from build123d import *

# Parameters (mm, degrees)
SALIENTE_EXTRUIR2_DEPTH      = 4.6
SALIENTE_EXTRUIR3_DEPTH      = 5.1
SALIENTE_EXTRUIR3_DEPTH_BACK = 4.6
CROQUIS2_R                   = 4.75
CROQUIS4_R                   = 5.025
SALIENTE_EXTRUIR4_DEPTH      = 1.5
CROQUIS6_R                   = 3.75
SALIENTE_EXTRUIR5_DEPTH      = 2.3
CROQUIS7_R                   = 4.5
SALIENTE_EXTRUIR6_DEPTH      = 2.8


with BuildPart() as part:
    # Croquis1 → Saliente-Extruir2 (new body)
    # profile 1 of 5: a face of its own
    with BuildSketch(Plane(origin=(0, 0, 0), x_dir=(1, 0, 0), z_dir=(0, 1, 0))):
        with BuildLine():
            ThreePointArc((6.5, 9.5), (8.621320344, 8.621320344), (9.5, 6.5))
            Line((9.5, 6.5), (9.5, -6.5))
            ThreePointArc((9.5, -6.5), (8.621320344, -8.621320344), (6.5, -9.5))
            Line((6.5, -9.5), (-6.5, -9.5))
            ThreePointArc((-6.5, -9.5), (-8.621320344, -8.621320344), (-9.5, -6.5))
            Line((-9.5, -6.5), (-9.5, 6.5))
            ThreePointArc((-9.5, 6.5), (-8.621320344, 8.621320344), (-6.5, 9.5))
            Line((-6.5, 9.5), (6.5, 9.5))
        make_face()
        with BuildLine():
            ThreePointArc((4.25, -4.75), (4.603553391, -4.603553391), (4.75, -4.25))
            Line((4.75, -4.25), (4.75, 4.25))
            ThreePointArc((4.75, 4.25), (4.603553391, 4.603553391), (4.25, 4.75))
            Line((4.25, 4.75), (-4.25, 4.75))
            ThreePointArc((-4.25, 4.75), (-4.603553391, 4.603553391), (-4.75, 4.25))
            Line((-4.75, 4.25), (-4.75, -4.25))
            ThreePointArc((-4.75, -4.25), (-4.603553391, -4.603553391), (-4.25, -4.75))
            Line((-4.25, -4.75), (4.25, -4.75))
        make_face(mode=Mode.SUBTRACT)
    # profile 2 of 5: a face of its own
    with BuildSketch(Plane(origin=(0, 0, 0), x_dir=(1, 0, 0), z_dir=(0, 1, 0))):
        with BuildLine():
            ThreePointArc((0, -4.75), (-3.358757211, -3.358757211), (-4.75, 0))
            Line((-4.75, 0), (-4.75, -4.25))
            ThreePointArc((-4.75, -4.25), (-4.603553391, -4.603553391), (-4.25, -4.75))
            Line((-4.25, -4.75), (0, -4.75))
        make_face()
    # profile 3 of 5: a face of its own
    with BuildSketch(Plane(origin=(0, 0, 0), x_dir=(1, 0, 0), z_dir=(0, 1, 0))):
        with BuildLine():
            Line((4.75, -4.25), (4.75, 0))
            ThreePointArc((4.75, 0), (3.358757211, -3.358757211), (0, -4.75))
            Line((0, -4.75), (4.25, -4.75))
            ThreePointArc((4.25, -4.75), (4.603553391, -4.603553391), (4.75, -4.25))
        make_face()
    # profile 4 of 5: a face of its own
    with BuildSketch(Plane(origin=(0, 0, 0), x_dir=(1, 0, 0), z_dir=(0, 1, 0))):
        with BuildLine():
            Line((4.25, 4.75), (0, 4.75))
            ThreePointArc((0, 4.75), (3.358757211, 3.358757211), (4.75, 0))
            Line((4.75, 0), (4.75, 4.25))
            ThreePointArc((4.75, 4.25), (4.603553391, 4.603553391), (4.25, 4.75))
        make_face()
    # profile 5 of 5: a face of its own
    with BuildSketch(Plane(origin=(0, 0, 0), x_dir=(1, 0, 0), z_dir=(0, 1, 0))):
        with BuildLine():
            Line((0, 4.75), (-4.25, 4.75))
            ThreePointArc((-4.25, 4.75), (-4.603553391, 4.603553391), (-4.75, 4.25))
            Line((-4.75, 4.25), (-4.75, 0))
            ThreePointArc((-4.75, 0), (-3.358757211, 3.358757211), (0, 4.75))
        make_face()
    extrude(amount=SALIENTE_EXTRUIR2_DEPTH)

    # Croquis2 → Saliente-Extruir3 (add, two sides: drawn at the far end of the back side and taken through both)
    with BuildSketch(Plane(origin=(0, 4.6, 0), x_dir=(1, 0, 0), z_dir=(0, 1, 0)).offset(-SALIENTE_EXTRUIR3_DEPTH_BACK)):
        with Locations(Location((0, 0, 0), (0, 0, 270))):
            Circle(CROQUIS2_R)
    extrude(amount=SALIENTE_EXTRUIR3_DEPTH + SALIENTE_EXTRUIR3_DEPTH_BACK)

    # Croquis4 → Saliente-Extruir4 (add)
    with BuildSketch(Plane(origin=(0, 9.7, 0), x_dir=(1, 0, 0), z_dir=(0, 1, 0))):
        with Locations(Location((0, 0, 0), (0, 0, 270))):
            Circle(CROQUIS4_R)
    extrude(amount=SALIENTE_EXTRUIR4_DEPTH)

    # Croquis6 → Saliente-Extruir5 (add)
    with BuildSketch(Plane(origin=(0, 11.2, 0), x_dir=(1, 0, 0), z_dir=(0, 1, 0))):
        with Locations(Location((0, 0, 0), (0, 0, 270))):
            Circle(CROQUIS6_R)
    extrude(amount=SALIENTE_EXTRUIR5_DEPTH)

    # Croquis7 → Saliente-Extruir6 (add)
    with BuildSketch(Plane(origin=(0, 13.5, 0), x_dir=(1, 0, 0), z_dir=(0, 1, 0))):
        with Locations(Location((0, 0, 0), (0, 0, 270))):
            Circle(CROQUIS7_R)
    extrude(amount=SALIENTE_EXTRUIR6_DEPTH)


solid = part.part
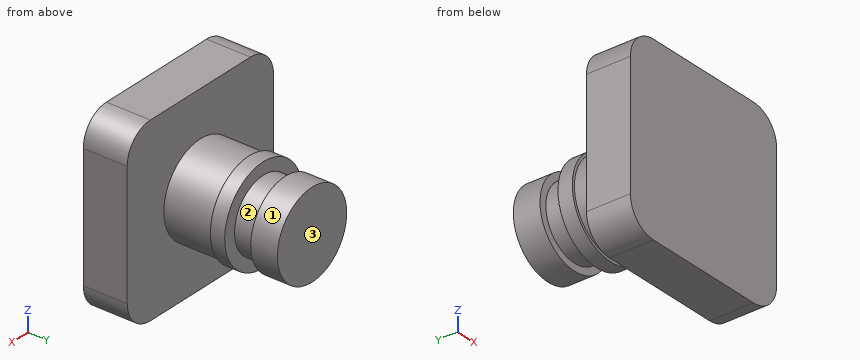
Geometry: final body of the model. Coordinates: model frame, mm. Face numbers are marked on the shaded views. A direction names the side the tool comes from. Give positions to 0.01 mm unless a question says otherwise; leave off trailing zeros. Write each loop counter-clockwise with the first axis right and the second up, starting at its lowest first coordinate (ties: lowest second). Pieces come first, ordered by that corner, then holes. Notation, with made-up numbers: (-29.5, 74.25) - (-19.5, 74.25) arc R19 ccw to (-19.5, 90.25) - close; hole circle Ø6 at (23, 73). An arc over 180 degrees is marked (long way). Return JSON: item names as keys, results as strings. Group by question number.
1) Set-up query: the marked faces 1, 2 and 3. Return all of +Z, -Z, +X, -X, +Y, -Y with unobstructed straight access to the full face (end or side cutting, diameter ignored); none if empty.
2) Line query: line 1 (Y direction, x = -3, z = -3.75); line 2 (Y direction, x = -3.5, z = 2.25); line 3 (Y direction, x = 2.25, z = 5.75). Output: solid intervals per line, ascending.
3) Section A-A on x = 0. Return the cut outline in (y, z) (3 decimals).
4) First-contact query: P1, Ø8, axis at x = -7.5, z = -7, coming from the +Y side; P2, Ø1.5, axis at y = 11, z = 2.5, coming from the +X side; P3, Ø2, axis at x = 5, y = 11.5, coming from the -Z side. Flat tips, straight axial feed; report the tip coordinate or a pass-through.
5) Section B-B on z = 0. Return the cut outline in (x, y) (3 decimals).
6) Section C-C on y = 6.25. Return the cut outline in (x, z), plus the area to 3 significant figures.
7) Section D-D on z = 8.5. Return the cut outline in (x, y), plus the area to 3 significant figures.
Filled in:
{
 "1": {"face 1": "+Y", "face 2": "none", "face 3": "+Z, -Z, +X, -X, +Y"},
 "2": {"line 1": "y = 0 to 4.6, 9.7 to 11.2", "line 2": "y = 0 to 11.2, 13.5 to 16.3", "line 3": "y = 0 to 4.6"},
 "3": {"outline": "(0, -9.5) - (4.6, -9.5) - (4.6, -4.75) - (9.7, -4.75) - (9.7, -5.025) - (11.2, -5.025) - (11.2, -3.75) - (13.5, -3.75) - (13.5, -4.5) - (16.3, -4.5) - (16.3, 4.5) - (13.5, 4.5) - (13.5, 3.75) - (11.2, 3.75) - (11.2, 5.025) - (9.7, 5.025) - (9.7, 4.75) - (4.6, 4.75) - (4.6, 9.5) - (0, 9.5) - close"},
 "4": {"P1": "stops at y = 4.6", "P2": "stops at x = 4.71", "P3": "stops at z = -2.98"},
 "5": {"outline": "(-9.5, 0) - (9.5, 0) - (9.5, 4.6) - (4.75, 4.6) - (4.75, 9.7) - (5.025, 9.7) - (5.025, 11.2) - (3.75, 11.2) - (3.75, 13.5) - (4.5, 13.5) - (4.5, 16.3) - (-4.5, 16.3) - (-4.5, 13.5) - (-3.75, 13.5) - (-3.75, 11.2) - (-5.025, 11.2) - (-5.025, 9.7) - (-4.75, 9.7) - (-4.75, 4.6) - (-9.5, 4.6) - close"},
 "6": {"outline": "circle Ø9.5 at (0, 0)", "area": "70.9 mm^2"},
 "7": {"outline": "(-8.74, 0) - (8.74, 0) - (8.74, 4.6) - (-8.74, 4.6) - close", "area": "80.4 mm^2"}
}
